```python
from build123d import *

# Parameters (mm, degrees)
SKETCH1_R          = 1.984375
BASE_EXTRUDE_DEPTH = 15.24
SKETCH3_R          = 2.794
EXTRUDE1_DEPTH     = 3.429


with BuildPart() as part:
    # Sketch1 → Base-Extrude (new body)
    with BuildSketch(Plane.XY):
        Circle(SKETCH1_R)
    extrude(amount=BASE_EXTRUDE_DEPTH)

    # Sketch2 → Boss-Revolve1 (revolve)
    with BuildSketch(Plane(origin=(0, 0, 0), x_dir=(1, 0, 0), z_dir=(0, 1, 0))):
        with BuildLine():
            Line((0, 1.7018), (0, 0))
            Line((0, 0), (3.96875, 0))
            ThreePointArc((3.96875, 0), (2.15911439, 1.258407907), (0, 1.7018))
        make_face()
    revolve(axis=Axis((0, 0, 0), (0, 0, -1)))

    # Sketch3 → Extrude1 (add)
    with BuildSketch(Plane.XY.offset(15.24)):
        Circle(SKETCH3_R)
    extrude(amount=-EXTRUDE1_DEPTH)


solid = part.part
```
CAD build for the part. Positions are in the model's coordinates, mm. Give positions to 0.01 mm unless a question says otherwise; leave off trailing zeros. Order: outer loops, then holes, each group sorted by start corner. A loop starts at its lowest first (then second) coordinate and runs counter-clockwise, first axis right, second up.
(1) Saw through at A-A, the plane y = 0. Give the cut face in (x, z), then the cut area to 3 significant figures.
(2) Saw through at D-D, the plane z = 4.25. Give the cut face in (x, y), then the cut area to 3 significant figures.
(3) Mould opens along Z. For faces 1 (the cylindrical face through (-2.217, -1.7, 13.55)), 2 (the flat face through (-1, -2, 0)), 3 (the flat face through (0, 0, 15.24)) say: released by +Z, released by -Z, zero draft, split by the parting line, or undercut.
(4) Saw through at B-B, the plane x = -1. Give the cut face in (y, z).
(5) Saw through at C-C, the plane x = 2.5. Give the cut face in (y, z), then the cut area to 3 significant figures.
(6) Drill centre lines: L1, parallel to Z at x = 2.5, y = 1; L2, parallel to Z at x = -2.25, y = 0; L3, parallel to Y at x = 0, z = 0.5. Where is each one in solid material? Low to high.
(7) Flat gauge pins, fed straight in: pin 1 (3 mm diameter, centred on x = 0.5, y = 0.5, fed in from -Z); pin 2 (3 mm diameter, centred on y = 2.5, z = 4, fed in from -X); pin 3 (1.5 mm diameter, centred on y = 2, z = 11, fed in from +X); pin 4 (4 mm diameter, centred on y = 1, z = 9, fed in from -X). Where does each tip first touch, or does it go through?
Results found:
1. outline: (-3.97, 0) arc R5.48 ccw to (3.97, 0) - (1.98, 0) - (1.98, 11.81) - (2.79, 11.81) - (2.79, 15.24) - (-2.79, 15.24) - (-2.79, 11.81) - (-1.98, 11.81) - (-1.98, 0) - close
1. area: 75.4 mm2
2. outline: circle Ø3.97 at (0, 0)
2. area: 12.4 mm2
3. face 1: zero draft
3. face 2: undercut
3. face 3: released by +Z
4. outline: (-3.84, 0) arc R5.39 ccw to (3.84, 0) - (1.71, 0) - (1.71, 11.81) - (2.61, 11.81) - (2.61, 15.24) - (-2.61, 15.24) - (-2.61, 11.81) - (-1.71, 11.81) - (-1.71, 0) - close
5. outline: (-3.08, 0) arc R4.87 ccw to (3.08, 0) - close; (-1.25, 11.81) - (1.25, 11.81) - (1.25, 15.24) - (-1.25, 15.24) - close
5. area: 13.2 mm2
6. L1: z = -0.99 to 0, 11.81 to 15.24
6. L2: z = -1.22 to 0, 11.81 to 15.24
6. L3: y = -1.98 to 1.98
7. pin 1: stops at z = -1.7
7. pin 2: stops at x = -1.71
7. pin 3: stops at x = 1.54
7. pin 4: stops at x = -1.98
